Here's how the part is built. I have some questions about the finished solid (model axes, mm). A direction names the side the tool comes from. Give positions to 0.01 mm unless a question says otherwise; leave off trailing zeros. Write each loop counter-clockwise with the first axis right and the second up, starting at its lowest first coordinate (ties: lowest second). Pieces come first, ordered by that corner, then holes. Notation, with made-up numbers: (-28, -8.5) - (13, -8.5) arc R12 cw to (13, 10.5) - close; hole circle Ø9 at (83.25, 24.25). An arc over 180 degrees is marked (long way). Use a Markdown table: item, result.
```python
from build123d import *

# Parameters (mm, degrees)
BOSS_EXTRUDE4_DEPTH       = 1.5875
M3_CLEARANCE_HOLE3_D      = 3
M3_CLEARANCE_HOLE1_D      = 3.1
M3_CLEARANCE_HOLE4_D      = 2.95
M3_CLEARANCE_HOLE2_D      = 3.1
M3_CLEARANCE_HOLE5_D      = 3
BOSS_EXTRUDE6_DEPTH       = 3.175
FILLET1_R                 = 2
FILLET3_R                 = 1
ALIGNMENT_CUTOUT_FL_DEPTH = 121.250075508
ALIGNMENT_CUTOUT_FR_DEPTH = 121.250075508
ALIGNMENT_CUTOUT_RL_DEPTH = 121.250075508
ALIGNMENT_CUTOUT_RR_DEPTH = 121.250075508


with BuildPart() as part:
    # Sketch1 → Boss-Extrude4 (new, symmetric)
    with BuildSketch(Plane(origin=(0, 0, 0), x_dir=(1, 0, 0), z_dir=(0, 1, 0))):
        with BuildLine():
            Line((-62.799553621, 32.496136604), (-73.969425011, 32.691107434))
            Line((-73.969425011, 32.691107434), (-77.053684287, 35.88495141))
            ThreePointArc((-77.053684287, 35.88495141), (-84.36642289, 10.358894189), (-83.446216027, -16.178041625))
            Line((-83.446216027, -16.178041625), (-79.680911643, -13.825218315))
            Line((-79.680911643, -13.825218315), (-69.484649137, -16.179210996))
            Line((-69.484649137, -16.179210996), (-43.894490772, -57.132025032))
            Line((-43.894490772, -57.132025032), (-43.894490772, -64.826600275))
            Line((-43.894490772, -64.826600275), (-43.094490772, -64.826600275))
            Line((-43.094490772, -64.826600275), (-34, -64.826600275))
            Line((-34, -64.826600275), (-34, -55.55))
            Line((-34, -55.55), (-34, -53.55))
            Line((-34, -53.55), (-20, -53.55))
            Line((-20, -53.55), (-19.718918331, -55.55))
            Line((-19.718918331, -55.55), (19.718918331, -55.55))
            Line((19.718918331, -55.55), (20, -53.55))
            Line((20, -53.55), (34, -53.55))
            Line((34, -53.55), (34, -55.55))
            Line((34, -55.55), (34, -64.826600275))
            Line((34, -64.826600275), (43.094490772, -64.826600275))
            Line((43.094490772, -64.826600275), (43.894490772, -64.826600275))
            Line((43.894490772, -64.826600275), (43.894490772, -57.132025032))
            Line((43.894490772, -57.132025032), (69.484649137, -16.179210996))
            Line((69.484649137, -16.179210996), (79.680911643, -13.825218315))
            Line((79.680911643, -13.825218315), (83.446216027, -16.178041625))
            ThreePointArc((83.446216027, -16.178041625), (84.610662337, -8.126242604), (85, 0))
            ThreePointArc((85, 0), (82.98964744, 18.377116688), (77.053684287, 35.88495141))
            Line((77.053684287, 35.88495141), (73.969425011, 32.691107434))
            Line((73.969425011, 32.691107434), (62.799553621, 32.496136604))
            Line((62.799553621, 32.496136604), (30.284668021, 63.895396642))
            Line((30.284668021, 63.895396642), (30.089697191, 75.065268032))
            Line((30.089697191, 75.065268032), (33.173956467, 78.259112008))
            ThreePointArc((33.173956467, 78.259112008), (0, 85), (-33.173956467, 78.259112008))
            Line((-33.173956467, 78.259112008), (-30.089697191, 75.065268032))
            Line((-30.089697191, 75.065268032), (-30.284668021, 63.895396642))
            Line((-30.284668021, 63.895396642), (-62.799553621, 32.496136604))
        make_face()
    extrude(amount=BOSS_EXTRUDE4_DEPTH, both=True)

    # M3 Clearance Hole3 (through all)
    with Locations(Plane(origin=(0, -1.5875, 0), x_dir=(-1, 0, 0), z_dir=(0, -1, 0))):
        with Locations((36.5, -50), (36.5, -38), (-36.5, -50), (-36.5, -38)):
            Hole(M3_CLEARANCE_HOLE3_D / 2)

    # M3 Clearance Hole1 (through all)
    with Locations(Plane(origin=(0, 1.5875, 0), x_dir=(1, 0, 0), z_dir=(0, 1, 0))):
        with Locations((-78.542321426, -8.49139241), (78.542321426, -8.49139241), (74.155025063, 27.240269049), (-74.155025063, 27.240269049)):
            Hole(M3_CLEARANCE_HOLE1_D / 2)

    # M3 Clearance Hole4 (through all)
    with Locations(Plane(origin=(0, -1.5875, 0), x_dir=(-1, 0, 0), z_dir=(0, -1, 0))):
        with Locations((-67.099301622, -15.278865202), (-50.141885166, -42.416404279), (-61.062544382, 30.698137949), (-38.043670771, 52.927205804), (50.141885166, -42.416404279), (67.099301622, -15.278865202), (38.043670771, 52.927205804), (61.062544382, 30.698137949)):
            Hole(M3_CLEARANCE_HOLE4_D / 2)

    # M3 Clearance Hole2 (through all)
    with Locations(Plane(origin=(0, 1.5875, 0), x_dir=(1, 0, 0), z_dir=(0, 1, 0))):
        with Locations((27, 76.497766718), (-27, 76.497766718)):
            Hole(M3_CLEARANCE_HOLE2_D / 2)

    # M3 Clearance Hole5 (through all)
    with Locations(Plane(origin=(0, 1.5875, 0), x_dir=(1, 0, 0), z_dir=(0, 1, 0))):
        with Locations((-11, -4.4), (11, -4.4), (11, -36.4), (-11, -36.4), (-11, 37.6), (11, 37.6)):
            Hole(M3_CLEARANCE_HOLE5_D / 2)

    # Sketch22 → Boss-Extrude6 (add)
    with BuildSketch(Plane(origin=(0, 1.5875, 0), x_dir=(1, 0, 0), z_dir=(0, 1, 0))):
        Polygon((65.061950694, 32.535626892), (30.245177733, 66.157793715), (30.284668021, 63.895396642), (62.799553621, 32.496136604), align=None)
        Polygon((-30.284668021, 63.895396642), (-30.245177733, 66.157793715), (-65.061950694, 32.535626892), (-62.799553621, 32.496136604), align=None)
        Polygon((43.894490772, -60.151352895), (71.689396914, -15.670204865), (69.484649137, -16.179210996), (43.894490772, -57.132025032), align=None)
        Polygon((-69.484649137, -16.179210996), (-71.689396914, -15.670204865), (-43.894490772, -60.151352895), (-43.894490772, -57.132025032), align=None)
    extrude(amount=-BOSS_EXTRUDE6_DEPTH)

    # Fillet1
    fillet1_edges = [part.edges().sort_by_distance(p)[0] for p in [
        (-30.245177733, -0.79375, -66.157793715),
        (-65.061950694, -0.79375, -32.535626892),
        (-71.689396914, 0.79375, 15.670204865),
        (-43.894490772, 0.79375, 60.151352895),
        (43.894490772, -0.79375, 60.151352895),
        (71.689396914, -0.79375, 15.670204865),
        (65.061950694, -0.79375, -32.535626892),
        (30.245177733, 0.79375, -66.157793715),
        (30.089697191, -0.79375, -75.065268032),
        (73.969425011, -0.79375, -32.691107434),
        (79.680911643, -0.79375, 13.825218315),
        (-79.680911643, -0.79375, 13.825218315),
        (-73.969425011, -0.79375, -32.691107434),
        (-30.089697191, -0.79375, -75.065268032),
    ]]
    fillet(fillet1_edges, radius=FILLET1_R)

    # Fillet3
    fillet3_edges = [part.edges().sort_by_distance(p)[0] for p in [
        (33.173956467, -0.79375, -78.259112008),
        (77.053684287, 0.79375, -35.88495141),
        (83.446216027, -0.79375, 16.178041625),
        (43.894490772, -0.79375, 64.826600275),
        (34, 0.79375, 64.826600275),
        (34, -0.79375, 53.55),
        (20, -0.79375, 53.55),
        (19.718918331, 0.79375, 55.55),
        (-19.718918331, 0.79375, 55.55),
        (-20, -0.79375, 53.55),
        (-34, -0.79375, 53.55),
        (-34, 0.79375, 64.826600275),
        (-43.894490772, -0.79375, 64.826600275),
        (-83.446216027, -0.79375, 16.178041625),
        (-77.053684287, -0.79375, -35.88495141),
        (-33.173956467, -0.79375, -78.259112008),
    ]]
    fillet(fillet3_edges, radius=FILLET3_R)

    # Sketch27 → Alignment Cutout - FL (cut, through all)
    with BuildSketch(Plane(origin=(0, 1.5875, 0), x_dir=(1, 0, 0), z_dir=(0, 1, 0))):
        Polygon((51.095385295, -37.11632527), (54.48757768, -39.236002327), (66.145801493, -20.578944211), (62.753609108, -18.459267154), align=None)
    extrude(amount=-ALIGNMENT_CUTOUT_FL_DEPTH, mode=Mode.SUBTRACT)

    # Sketch28 → Alignment Cutout - FR (cut, through all)
    with BuildSketch(Plane(origin=(0, 1.5875, 0), x_dir=(1, 0, 0), z_dir=(0, 1, 0))):
        Polygon((-54.48757768, -39.236002327), (-51.095385295, -37.11632527), (-62.753609108, -18.459267154), (-66.145801493, -20.578944211), align=None)
    extrude(amount=-ALIGNMENT_CUTOUT_FR_DEPTH, mode=Mode.SUBTRACT)

    # Sketch29 → Alignment Cutout - RL (cut, through all)
    with BuildSketch(Plane(origin=(0, 1.5875, 0), x_dir=(1, 0, 0), z_dir=(0, 1, 0))):
        Polygon((40.251053032, 48.015234351), (43.029686514, 50.892593553), (58.855162121, 35.610109402), (56.07652864, 32.732750201), align=None)
    extrude(amount=-ALIGNMENT_CUTOUT_RL_DEPTH, mode=Mode.SUBTRACT)

    # Sketch30 → Alignment Cutout - RR (cut, through all)
    with BuildSketch(Plane(origin=(0, 1.5875, 0), x_dir=(1, 0, 0), z_dir=(0, 1, 0))):
        Polygon((-56.07652864, 32.732750201), (-58.855162121, 35.610109402), (-43.029686514, 50.892593553), (-40.251053032, 48.015234351), align=None)
    extrude(amount=-ALIGNMENT_CUTOUT_RR_DEPTH, mode=Mode.SUBTRACT)


solid = part.part
```
Item 1: Will these pins go through, and if not, where does the flat tip stop? pin 1 Ø3.5 at (x, z) = (-67.1, 15.28) entering from -Y; pin 2 Ø1.6 at (y, z) = (0.5, 57.5) entering from -X.
Values:
| item | result |
|---|---|
| pin 1 | stops at y = -1.59 |
| pin 2 | stops at x = -46.05 |
Item 2: If we section it at A-A, the plane y = 0.1: Count the separate pieces of the cut face and the enclosed holes in it, plus the area to 3 significant figures.
Values:
| item | result |
|---|---|
| separate pieces | 1 |
| enclosed holes | 28 |
| area | 16,600 mm2 |
Item 3: For faces 1 (the cylindrical face through (84.41, 0.02, -10.01)), 2 (the flat face through (-60.398, 0.022, 29.777)), which set-ups out of +Z, -Z, +X, -X, +Y, -Y let a thin tool reach every point of the face, with its end or its side?
Values:
| item | result |
|---|---|
| face 1 | +X, +Y, -Y |
| face 2 | +Y, -Y |
Item 4: If we section it at B-B, the plane z = -15: Write out the boundary of the cut face in (x, y), plus the area to 3 significant figures.
Values:
| item | result |
|---|---|
| outline | (-83.67, -1.59) - (83.67, -1.59) - (83.67, 1.59) - (-83.67, 1.59) - close |
| area | 531 mm2 |
Item 5: Thinking about a two-plate mould opening in Z: for faces 3 (the flat face through (-56.84, 0.02, 27.92)), 4 (the cylindrical face through (-84.323, 0.022, -10.709)), 5 (the flat face through (-1, -1.588, -11)), 6 (the flat face through (57.535, 0.022, 38.322)), which applies, +Z half, -Z half, draft (parallel to the pull), parting line (faces both ways), or undercut?
Values:
| item | result |
|---|---|
| face 3 | undercut |
| face 4 | parting line |
| face 5 | draft |
| face 6 | +Z half |
Item 6: I need wall thicknesses on line 1 along X through (y, z) = (0.9, -76.5); line 2 along X through (y, z) = (-0.8, -47); line 3 along Z through (x, y) = (59.5, 0.95). Which ranges of each line are inside material? Lowest first, please. Write a range as [from, to].
Values:
| item | result |
|---|---|
| line 1 | x = [-31.48, -28.55], [-25.45, 25.45], [28.55, 31.48] |
| line 2 | x = [-50.08, -47.06], [-41.3, 41.3], [47.06, 50.08] |
| line 3 | z = [-37.91, 23.67], [31.21, 35.18] |
